The model under review builds one solid part; all positions refer to its coordinate system, in mm. A direction names the side the tool comes from. Round coordinates to 2 decimals unless told otherwise and drop trailing zeros. Use a Markdown table: item, result. Add a question column.
1) Insertion check: pin 1 (1.8 mm diameter, centred on y = 15, z = 30, fed in from +X). The pin has a flat end and moves straight along its axis. Give the tip position at first contact, or say it passes through.
2) For faces 4 (the flat face through (34.5, 15, 2)), 5 (the flat face through (1, 0, 0)), list the 3-axis set-ups (+Z, -Z, +X, -X, +Y, -Y) from which the entire face can be reached by the end or side of a thin tool; tool diameter is ignored.
3) Wall thickness on probe 1 along Y at (x, z) = (35.75, 2): over which ranges is the line inside the solid? List them lowest first.
4) Mouldability with a two-part tool opening along Y and no side actions: class faces 1 (the flat face through (-1, 13, 35)), 2 (the flat face through (1, 27, 0)), 3 (the flat face through (34.5, 15, 30)) as released by +Y, released by -Y, zero draft, split by the parting line, or undercut.
Autodesk Inventor part; units mm, degrees
ref_plane "YZ Plane" through (0, 0, 0) normal (1, 0, 0) x (0, 1, 0)
ref_plane "XZ Plane" through (0, 0, 0) normal (0, 1, 0) x (-1, 0, 0)
ref_plane "XY Plane" through (0, 0, 0) normal (0, 0, 1) x (1, 0, 0)
sketch "Sketch1" plane through (0, 0, 0) normal (0, 1, 0) x (-1, 0, 0)
  line L0 (37.5, 35) -> (-37.5, 35)
  line L1 (-37.5, 35) -> (-37.5, -35)
  line L2 (-37.5, -35) -> (37.5, -35)
  line L3 (37.5, -35) -> (37.5, 35)
  point P0 (0, 0)
  point P1 (37.5, 0)
  point P2 (0, -35)
  dimension "d1" = 75
  dimension "d2" = 70
extrude "Extrusion1" add sketch "Sketch1" along normal blind 27
sketch "Sketch2" plane through (37.5, 0, 35) normal (1, 0, 0) x (0, 0, -1)
  circle A0 centre (5, 15) radius 1.5
  line L0 (0, 27) -> (70, 27)
  line L1 (0, 0) -> (0, 27)
  circle A1 centre (33, 15) radius 1.5
  point P0 (35, 0)
  dimension "d5" = 3
  dimension "d6" = 12
  dimension "d7" = 5
  dimension "d8" = 3
  dimension "d9" = 28
extrude "Extrusion2" cut sketch "Sketch2" against normal blind 3
equation "\"d8\" = d5"
properties part number "power_supply"
Result set:
| question | item | result |
|---|---|---|
| 1 | pin 1 | x = 34.5 |
| 2 | face 4 | +X |
| 2 | face 5 | +Z, -Z, +X, -X, -Y |
| 3 | probe 1 | 0 to 13.5, 16.5 to 27 |
| 4 | face 1 | zero draft |
| 4 | face 2 | released by +Y |
| 4 | face 3 | undercut |
